Could you check a few things on this drawing? It's one solid part, dimensions in mm from its lowest x, y, z. Give positions to 0.01 mm unless a question says otherwise; leave off trailing zeros. Order: outer loops, then holes, each group sorted by start corner. A loop starts at its lowest first (then second) coordinate and runs counter-clockwise, first axis right, second up.
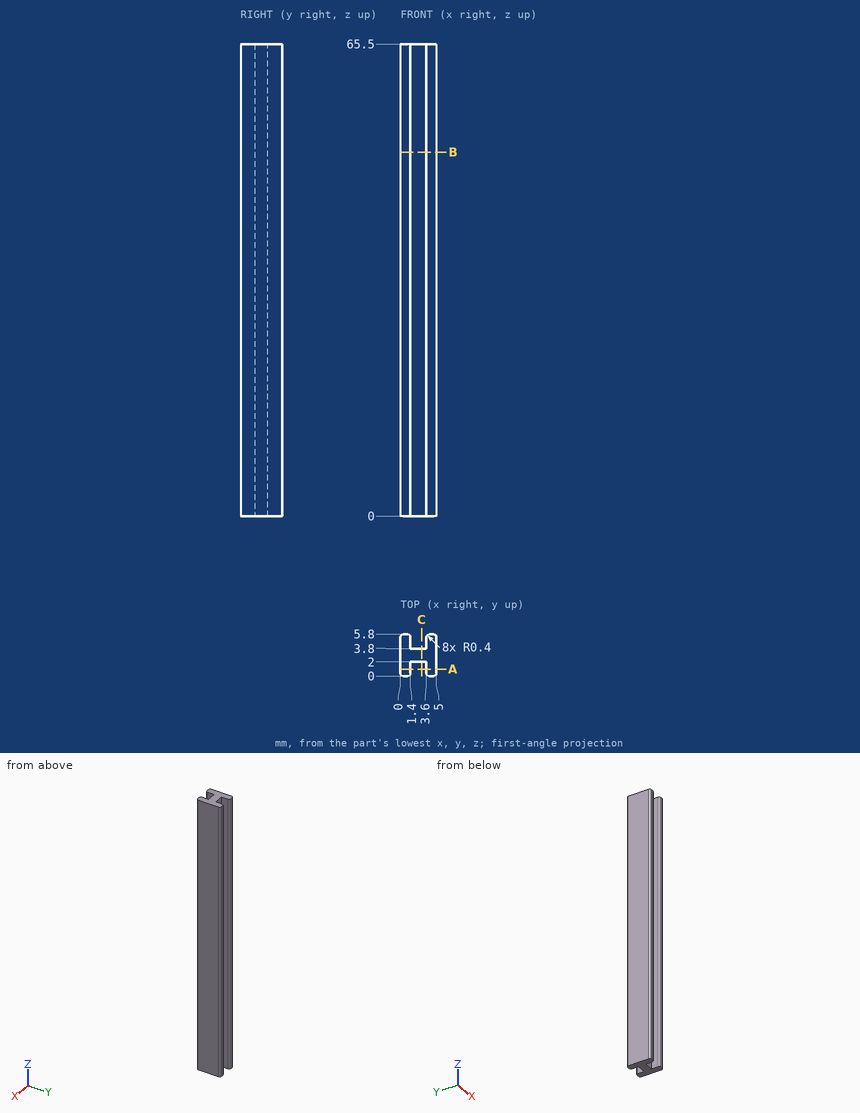
Item 1: Imagine slicing it at A-A on y = 0.95. List the corners of the cut face in (x, z) for me.
Findings:
outline: (0, 0) - (1.4, 0) - (1.4, 65.5) - (0, 65.5) - close; (3.6, 0) - (5, 0) - (5, 65.5) - (3.6, 65.5) - close
Item 2: Please list where these lines run through material, in increasing order: line 1 along X through (y, z) = (1.8, 14); line 2 along Y through (x, z) = (1.8, 14); line 3 along Y through (x, z) = (0.3, 26.5).
Findings:
line 1: x = 0 to 1.4, 3.6 to 5
line 2: y = 2 to 3.8
line 3: y = 0.01 to 5.79
Item 3: Imagine slicing it at C-C on x = 2.95. List the corners of the cut face in (y, z) for me, then the cut area to 3 significant figures.
Findings:
outline: (2, 0) - (3.8, 0) - (3.8, 65.5) - (2, 65.5) - close
area: 118 mm2
Item 4: For pin 1 (2 mm diameter, centred on x = 2.5, z = 37.5, fed in from -Y), with a flat end and sliding along its axis, tell me the tip position at first contact or that it passes through.
Findings:
pin 1: stops at y = 2
Item 5: Imagine slicing it at B-B on z = 50.5. List the corners of the cut face in (x, y) for me, then the cut area to 3 significant figures.
Findings:
outline: (0, 0.4) arc R0.4 ccw to (0.4, 0) - (1, 0) arc R0.4 ccw to (1.4, 0.4) - (1.4, 2) - (3.6, 2) - (3.6, 0.4) arc R0.4 ccw to (4, 0) - (4.6, 0) arc R0.4 ccw to (5, 0.4) - (5, 5.4) arc R0.4 ccw to (4.6, 5.8) - (4, 5.8) arc R0.4 ccw to (3.6, 5.4) - (3.6, 3.8) - (1.4, 3.8) - (1.4, 5.4) arc R0.4 ccw to (1, 5.8) - (0.4, 5.8) arc R0.4 ccw to (0, 5.4) - close
area: 19.9 mm2
